Design review of the part built by this model. Coordinates are the model's own, in mm. Coordinates: 2 decimals unless noted, no trailing zeros. Loops run counter-clockwise (first coordinate to the right, second up) from the corner with the lowest first, then second, coordinate; pieces in that order, holes last.
Q1. Wall thickness on probe 1 along Z at (x, y) = (-17.5, -24.5); probe 2 along Y at (x, z) = (-39.2, 4); probe 3 along X at (y, z) = (-27, 4.5): over which ranges is each line inside the solid? List them lowest first.
Q2. For P1, Ø2, axis at y = -22.24, z = 4, coming from the +X side; P2, Ø2, axis at x = -28, y = -13.5, coming from the +Z side; P3, Ø1.2, axis at y = -22.5, z = 3.5, coming from the -X side, all flat-tipped, find the tip position at first contact; note any pin that passes through.
Q3. Add section C-C on y = -17.5. Give the boundary of the cut face in (x, z), and give its area (3 significant figures).
Q4. Add section D-D on z = 6. Give the boundary of the cut face in (x, y), and give its area (3 significant figures).
Q5. Add section B-B on x = -11.5. Give the boundary of the cut face in (y, z), and give its area (3 significant figures).
Q6. Add section A-A on z = 3.25. Give the boundary of the cut face in (x, y), and give its area (3 significant figures).
```python
from build123d import *

# Parameters (mm, degrees)
EXTRUDE_2_DEPTH        = 8
HOLE_WIZARD_M3_1_D     = 2.5
HOLE_WIZARD_M3_1_DEPTH = 5
HOLE_WIZARD_M3_2_D     = 2.5
HOLE_WIZARD_M3_2_DEPTH = 5


with BuildPart() as part:
    # 草图1 → 凸台-拉伸2 (new body)
    with BuildSketch(Plane.XY):
        Polygon((-42.3029947, -7.235847593), (-42.3029947, -32.235847593), (0.998275489, -32.235847593), align=None)
    extrude(amount=EXTRUDE_2_DEPTH)

    # M3 螺纹孔1
    with Locations(Plane.ZY.offset(42.3029947)):
        with Locations((4, -22.235847593)):
            Hole(HOLE_WIZARD_M3_1_D / 2, depth=HOLE_WIZARD_M3_1_DEPTH)

    # M3 螺纹孔2
    with Locations(Plane(origin=(-13.708962592, -23.744619728, 0), x_dir=(0.8660254037844363, -0.5000000000000042, 0), z_dir=(0.5000000000000042, 0.8660254037844363, 0))):
        with Locations((-3.01754427, -4)):
            Hole(HOLE_WIZARD_M3_2_D / 2, depth=HOLE_WIZARD_M3_2_DEPTH)


solid = part.part
```
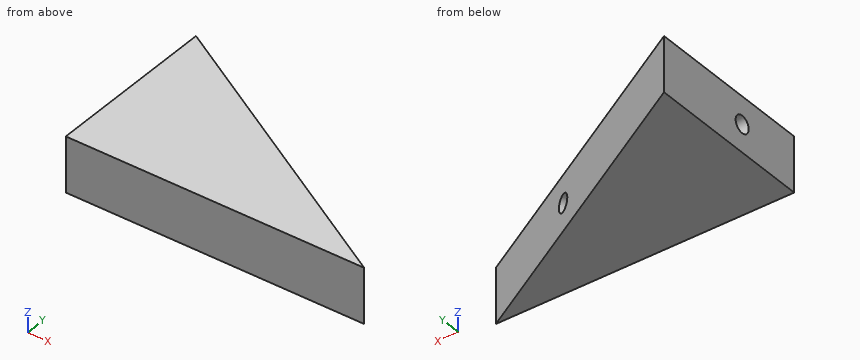
Entries:
1. probe 1: z = 0 to 2.76, 5.24 to 8
1. probe 2: y = -32.24 to -23.49, -20.99 to -9.03
1. probe 3: x = -42.3 to -18.07, -17.75 to -8.07
2. P1: stops at x = -14.58
2. P2: passes through
2. P3: stops at x = -37.3
3. outline: (-42.3, 0) - (-24.52, 0) - (-24.52, 8) - (-42.3, 8) - close
3. area: 142 mm2
4. outline: (-42.3, -32.24) - (1, -32.24) - (-42.3, -7.24) - close
4. area: 541 mm2
5. outline: (-32.24, 0) - (-25.02, 0) - (-25.02, 8) - (-32.24, 8) - close
5. area: 57.7 mm2
6. outline: (-42.3, -32.24) - (1, -32.24) - (-15.46, -22.74) - (-17.96, -27.07) - (-19.69, -26.07) - (-17.19, -21.74) - (-42.3, -7.24) - (-42.3, -21.24) - (-37.3, -21.24) - (-37.3, -23.24) - (-42.3, -23.24) - close
6. area: 521 mm2
